Answer from the drawing. Dimensions are ordinates in mm from the lowest x, y and z of the part. A direction names the side the tool comes from. Coordinates: 2 decimals unless noted, no trailing zeros. Order: outer loops, then holes, each group sorted by start corner. A loop starts at its lowest first (then second) coordinate and runs counter-clockwise, first axis right, second up.
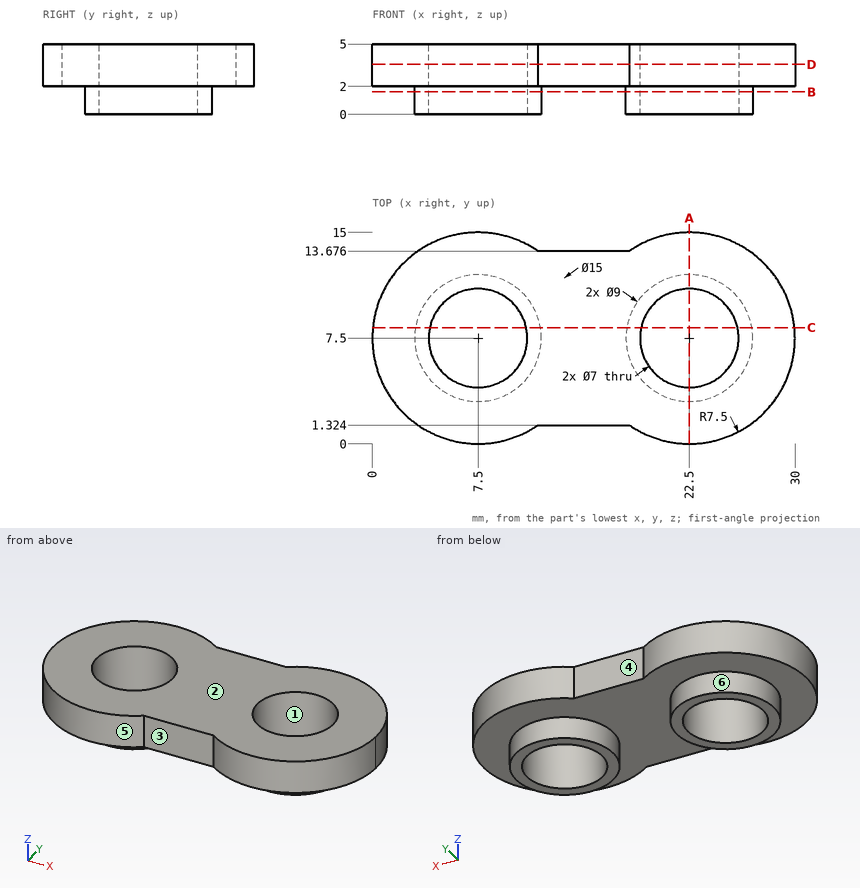
1) Section B-B (z = 1.6) is taken. Give the vertices of the cut face in (x, y).
2) Section A-A (x = 22.5) is taken. Give the vertices of the cut face in (y, z), then the cut area to 3 significant figures.
3) Each of these flat-tipped pins is pushed along its axis until it touches: P1, Ø0.9, axis at x = 16.5, z = 3, coming from the -Y side; P2, Ø4, axis at x = 8, y = 2, coming from the -Z side; P3, Ø1.5, axis at y = 4.5, z = 3, coming from the +X side (1 decimal); P4, Ø4.5, axis at x = 15.5, y = 11, coming from the -Z side. Where does it stop, or does it pass through?
4) Consider L1, parallel to Y at x = 7.5, z = 3.35; L2, parallel to X at y = 8, z = 1.5; L3, parallel to X at y = 6.5, z = 4. Determine where each line is inside the solid, lowest interval first.
5) Determine the mould class of the marked faces 1 and 2 for opening direction X: released by +X, released by -X, zero draft, split by the parting line, or undercut.
6) Section D-D (z = 3.55) is taken. Give the vertices of the cut face in (x, y), then the cut area to 3 significant figures.
7) A tool of negligible diameter and unlimited length cuts with its end or side. For the marked faces 3, 4, 5 and 6, from which of +Z, -Z, +X, -X, +Y, -Y can it reach the whole face along a straight path? Write none if from no direction.
8) Section C-C (y = 8.25) is taken. Give the vertices of the cut face in (x, z), then the cut area to 3 significant figures.
Filled sheet:
1. outline: circle Ø9 at (7.5, 7.5); circle Ø9 at (22.5, 7.5); hole circle Ø7 at (7.5, 7.5); hole circle Ø7 at (22.5, 7.5)
2. outline: (0, 2) - (3, 2) - (3, 0) - (4, 0) - (4, 5) - (0, 5) - close; (11, 0) - (12, 0) - (12, 2) - (15, 2) - (15, 5) - (11, 5) - close
2. area: 28.0 mm2
3. P1: stops at y = 1.32
3. P2: stops at z = 0
3. P3: stops at x = 29.7
3. P4: stops at z = 2
4. L1: y = 0 to 4, 11 to 15
4. L2: x = 3.03 to 4.04, 10.96 to 11.97, 18.03 to 19.04, 25.96 to 26.97
4. L3: x = 0.07 to 4.15, 10.85 to 19.15, 25.85 to 29.93
5. face 1: undercut
5. face 2: zero draft
6. outline: (11.76, 1.32) - (18.24, 1.32) arc R7.5 ccw to (30, 7.5) arc R7.5 ccw to (18.24, 13.68) - (11.76, 13.68) arc R7.5 ccw (long way) to start; hole circle Ø7 at (7.5, 7.5); hole circle Ø7 at (22.5, 7.5)
6. area: 300 mm2
7. face 3: +Z, -Z, -Y
7. face 4: +Z, -Z, +Y
7. face 5: +Z, -Z
7. face 6: -Z
8. outline: (0.04, 2) - (3.06, 2) - (3.06, 0) - (4.08, 0) - (4.08, 5) - (0.04, 5) - close; (10.92, 0) - (11.94, 0) - (11.94, 2) - (18.06, 2) - (18.06, 0) - (19.08, 0) - (19.08, 5) - (10.92, 5) - close; (25.92, 0) - (26.94, 0) - (26.94, 2) - (29.96, 2) - (29.96, 5) - (25.92, 5) - close
8. area: 56.9 mm2
